from build123d import *

# Parameters (mm, degrees)
CYLINDER_R              = 10
CYLINDER_DEPTH          = 10
CYLINDER001_R           = 2
CYLINDER001_DEPTH       = 30
PAD001_DEPTH            = 30
CYLINDER002_R           = 4
CYLINDER002_DEPTH       = 40
CYLINDER002_PITCH_ANGLE = 90
BOX003_W                = 8
BOX003_H                = 10
BOX003_DEPTH            = 10
BOX002_W                = 8
BOX002_H                = 10
BOX002_DEPTH            = 10
BOX001_W                = 4
BOX001_H                = 12
BOX001_DEPTH            = 10
BOX_W                   = 40
BOX_H                   = 35
BOX_DEPTH               = 10


with BuildPart() as cylinder:
    # Cylinder → Cylinder (new body)
    with BuildSketch(Plane.XY.offset(-5)):
        Circle(CYLINDER_R)
    extrude(amount=CYLINDER_DEPTH)


with BuildPart() as cylinder001:
    # Cylinder001 → Cylinder001 (new body)
    with BuildSketch(Plane(origin=(-15, -15, 0), x_dir=(0, -1, 0), z_dir=(1, 0, 0))):
        Circle(CYLINDER001_R)
    extrude(amount=CYLINDER001_DEPTH)


with BuildPart() as other_nut:
    # Sketch001 → Pad001 (new body)
    with BuildSketch(Plane.YZ):
        Polygon((3.464102, 6), (-3.464102, 6), (-6.928203, 0), (-3.464102, -6), (3.464102, -6), (6.928203, 0), align=None)
    extrude(amount=-PAD001_DEPTH)


with BuildPart() as other_nut_1:
    # Body001 placement: moved
    add(other_nut.part.moved(Location((15, 0, 0))))


with BuildPart() as other_screw:
    # Cylinder002 → Cylinder002 (new body)
    with BuildSketch(Plane.XY):
        Circle(CYLINDER002_R)
    extrude(amount=CYLINDER002_DEPTH)


with BuildPart() as other_screw_1:
    # Cylinder002 pitch: moved
    add(other_screw.part.rotate(Axis((0, 0, 0), (0, 1, 0)), CYLINDER002_PITCH_ANGLE))


with BuildPart() as other_screw_2:
    # Cylinder002 placement: moved
    add(other_screw_1.part.moved(Location((-20, 0, 0))))


with BuildPart() as cube003:
    # Box003 → Box003 (new body)
    with BuildSketch(Plane(origin=(-20, -20, -5), x_dir=(1, 0, 0), z_dir=(0, 0, 1))):
        with Locations((4, 5)):
            Rectangle(BOX003_W, BOX003_H)
    extrude(amount=BOX003_DEPTH)


with BuildPart() as cube002:
    # Box002 → Box002 (new body)
    with BuildSketch(Plane(origin=(12, -20, -5), x_dir=(1, 0, 0), z_dir=(0, 0, 1))):
        with Locations((4, 5)):
            Rectangle(BOX002_W, BOX002_H)
    extrude(amount=BOX002_DEPTH)


with BuildPart() as negative_fusion:
    # Box001 → Box001 (new body)
    with BuildSketch(Plane(origin=(-2, -20, -5), x_dir=(1, 0, 0), z_dir=(0, 0, 1))):
        with Locations((2, 6)):
            Rectangle(BOX001_W, BOX001_H)
    extrude(amount=BOX001_DEPTH)

    # Fusion: union Cylinder, Cylinder001, Other Nut, Other Screw, Cube003, Cube002
    add(cylinder.part)
    add(cylinder001.part)
    add(other_nut_1.part)
    add(other_screw_2.part)
    add(cube003.part)
    add(cube002.part)


with BuildPart() as cut:
    # Box → Box (new body)
    with BuildSketch(Plane(origin=(-20, -20, -5), x_dir=(1, 0, 0), z_dir=(0, 0, 1))):
        with Locations((20, 17.5)):
            Rectangle(BOX_W, BOX_H)
    extrude(amount=BOX_DEPTH)

    # Cut: cut Negative Fusion
    add(negative_fusion.part, mode=Mode.SUBTRACT)


solid = cut.part
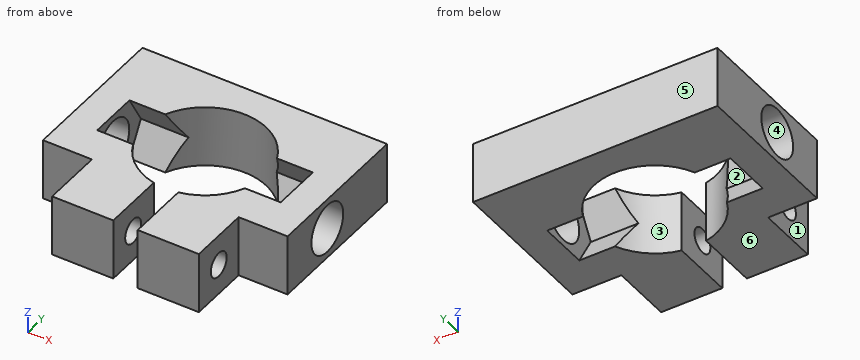
Geometry: final body of the model. Coordinates: model frame, mm. Face numbers are marked on the shaded views. A direction names the side the tool comes from. Round coordinates to 2 decimals unless told otherwise and drop trailing zeros. Loops run counter-clockwise (first coordinate to the right, second up) from the corner with the lowest first, then second, coordinate; pieces in that order, holes last. Notation, with made-up numbers: M 4.5,48.25 L 38.5,48.25 A17 ccw 38.5,52.25 Z; hole C 25.5,-6 d11. An arc over 180 degrees is marked long. Put each result on its own line as item: value. Start each with the question number.
(1) Draft query along Z for the marked faces 4, 5 and 6. Return one class per face: +Z half, -Z half, draft (parallel to the pull), parting line (faces both ways), or undercut.
(2) Section query B-B (x = -5.5). Return loops of the section in (y, z).
(3) Section query D-D (z = 3). Return loops of the section in (x, y).
(4) Section query C-C (y = -5.5). Return loops of the section in (x, z), then the cut area to 3 significant figures.
(5) Contact query for flat-ended pins moving along their axis: pin 1 Ø5 at (y, z) = (-15, 0) entering from -X; pin 2 Ø5 at (y, z) = (-14, 2) entering from +X; pin 3 Ø2.5 at (x, z) = (15, 1.5) entering from -Y. Output: stop coordinate, or through.
(6) Material intervals for line 1 along Z through (x, y) = (7, -15); line 2 along X through (y, z) = (-4, -1.75); line 3 along Y through (x, z) = (17.4, 0), sorted ascending. Write a range as [from, to].
(7) Section query A-A (y = 0). Return loops of the section in (x, z), then the cut area to 3 significant figures.
(8) Set-up query: the marked faces 1, 2 and 3. Return all of +Z, -Z, +X, -X, +Y, -Y with unobstructed straight access to the full face (end or side cutting, diameter ignored); none if empty.
Findings below:
1. face 4: undercut
1. face 5: draft
1. face 6: -Z half
2. outline: M -20,-5 L -8.35,-5 L -8.35,5 L -20,5 Z; M 8.35,-5 L 15,-5 L 15,5 L 8.35,5 Z; hole C -15,0 d4
3. outline: M -20,-10 L -12,-10 L -12,-20 L -2,-20 L -2,-9.8 A10 cw -8.54,-5.2 L -15,-5.2 L -15,-2.65 L -20,-2.65 Z; M -20,2.65 L -15,2.65 L -15,5.2 L -8.54,5.2 A10 cw 8.54,5.2 L 15,5.2 L 15,2.65 L 20,2.65 L 20,15 L -20,15 Z; M 2,-20 L 12,-20 L 12,-10 L 20,-10 L 20,-2.65 L 15,-2.65 L 15,-5.2 L 8.54,-5.2 A10 cw 2,-9.8 Z
4. outline: M -20,-5 L -8.35,-5 L -8.35,-2.47 L -15,-2.47 L -15,2.47 L -8.35,2.47 L -8.35,5 L -20,5 Z; M 8.35,-5 L 20,-5 L 20,5 L 8.35,5 L 8.35,2.47 L 15,2.47 L 15,-2.47 L 8.35,-2.47 Z
4. area: 167 mm2
5. pin 1: stops at x = -12
5. pin 2: stops at x = 12
5. pin 3: stops at y = -10
6. line 1: z = [-5, -2], [2, 5]
6. line 2: x = [-20, -15], [15, 20]
6. line 3: y = [-10, -4], [4, 15]
7. outline: M -20,-5 L -15,-5 L -15,-4 L -20,-4 Z; M -20,4 L -15,4 L -15,5 L -20,5 Z; M 15,-5 L 20,-5 L 20,-4 L 15,-4 Z; M 15,4 L 20,4 L 20,5 L 15,5 Z
7. area: 20.0 mm2
8. face 1: +Z, -Z, -X, -Y
8. face 2: none
8. face 3: +Z, -Z
